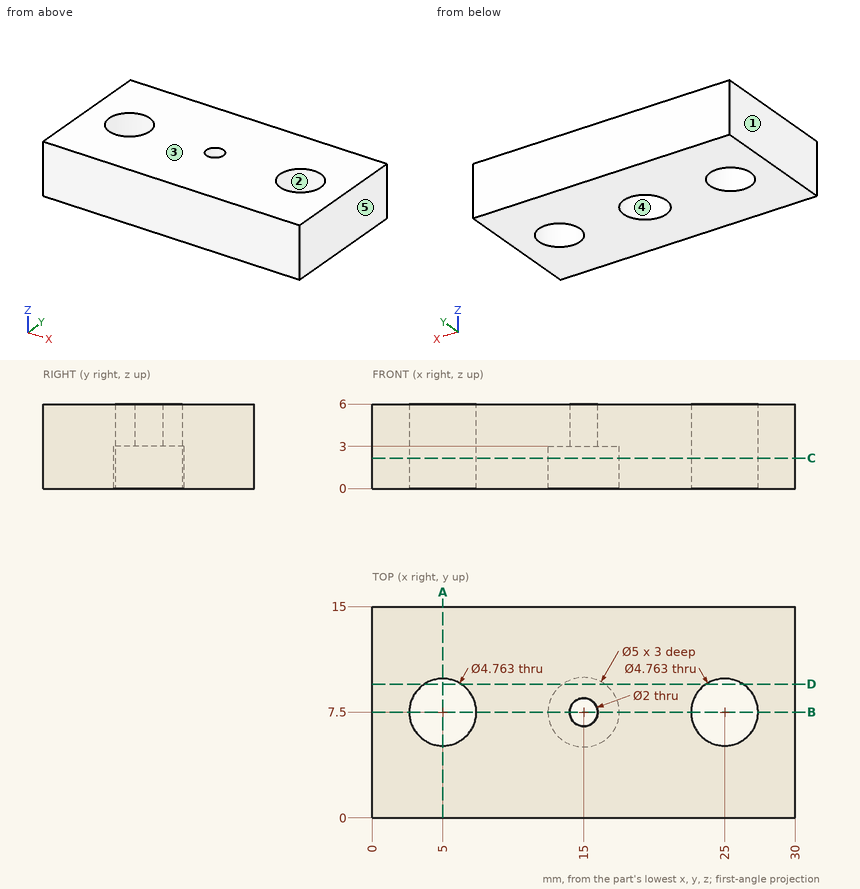
Study the drawing (mm; zero at the part's minimum x, y, z) and answer. A direction names the side the tool comes from. Give positions to 0.01 mm unless a question says otherwise; leave off trailing zeros. Order: outer loops, then holes, each group sorted by start corner. A loop starts at its lowest first (then second) coordinate and runs counter-clockwise, first axis right, second up. Notation, with made-up numbers: (6.5, 75.25) - (64.5, 75.25) arc R31 cw to (64.5, 99.25) - close; hole circle Ø3 at (27.5, 19). An arc over 180 degrees is marked (long way). Answer in a Markdown table with one row per item. Add a question column.
Q1. The part is cut by section B-B (y = 7.5). Determine the outline of the cut face in (x, z), then the cut area to 3 significant figures.
Q2. The part is cut by section A-A (x = 5). Determine the outline of the cut face in (y, z).
Q3. The part is cut by section C-C (z = 2.15). Determine the outline of the cut face in (x, y).
Q4. The part is cut by section D-D (y = 9.5). Determine the outline of the cut face in (x, z), then the cut area to 3 significant figures.
Q5. Given P1, Ø1.5, axis at x = 14, y = 8.5, coming from the -Z side; P2, Ø3, axis at x = 25, y = 7.5, coming from the -Z side; P3, Ø4, axis at x = 6.5, y = 13, coming from the -Z side, each flat-ended and moving along its own axis, determine where each tip first touches the part or whether it passes through.
Q6. Find the intervals of material crossed by line 1 along Y through (x, z) = (5, 1.3); line 2 along X through (y, z) = (5.5, 1.5) (1 decimal); line 3 along X through (y, z) = (7, 2.5), in increasing order. Write a range as [from, to].
Q7. For a pull along X with two mould halves and no side action, classify the marked faces 1, 2 and 3 as released by +X, released by -X, zero draft, split by the parting line, or undercut.
Q8. Which of the six approach directions +Z, -Z, +X, -X, +Y, -Y give full straight-line access (tool end or side, diameter ignored) to the marked faces 4 and 5?
Determined:
| question | item | result |
|---|---|---|
| 1 | outline | (0, 0) - (2.62, 0) - (2.62, 6) - (0, 6) - close; (7.38, 0) - (12.5, 0) - (12.5, 3) - (14, 3) - (14, 6) - (7.38, 6) - close; (16, 3) - (17.5, 3) - (17.5, 0) - (22.62, 0) - (22.62, 6) - (16, 6) - close; (27.38, 0) - (30, 0) - (30, 6) - (27.38, 6) - close |
| 1 | area | 102 mm² |
| 2 | outline | (0, 0) - (5.12, 0) - (5.12, 6) - (0, 6) - close; (9.88, 0) - (15, 0) - (15, 6) - (9.88, 6) - close |
| 3 | outline | (0, 0) - (30, 0) - (30, 15) - (0, 15) - close; hole circle Ø4.76 at (5, 7.5); hole circle Ø5 at (15, 7.5); hole circle Ø4.76 at (25, 7.5) |
| 4 | outline | (0, 0) - (3.71, 0) - (3.71, 6) - (0, 6) - close; (6.29, 0) - (13.5, 0) - (13.5, 3) - (16.5, 3) - (16.5, 0) - (23.71, 0) - (23.71, 6) - (6.29, 6) - close; (26.29, 0) - (30, 0) - (30, 6) - (26.29, 6) - close |
| 4 | area | 140 mm² |
| 5 | P1 | stops at z = 3 |
| 5 | P2 | passes through |
| 5 | P3 | stops at z = 0 |
| 6 | line 1 | y = [0, 5.12], [9.88, 15] |
| 6 | line 2 | x = [0, 3.7], [6.3, 13.5], [16.5, 23.7], [26.3, 30] |
| 6 | line 3 | x = [0, 2.67], [7.33, 12.55], [17.45, 22.67], [27.33, 30] |
| 7 | face 1 | released by -X |
| 7 | face 2 | undercut |
| 7 | face 3 | zero draft |
| 8 | face 4 | -Z |
| 8 | face 5 | +Z, -Z, +X, +Y, -Y |
